Solid Edge part; units mm, degrees
sketch "Sketch1" plane through (0, 0, 0) normal (1, 0, 0) x (0, 1, 0)
  line L0 (0, 0) -> (43.8289, 0)
sketch "Sketch2" plane through (0, 0, 0) normal (0, -1, 0) x (1, 0, 0)
  line L0 (0, 50.8) -> (0, 0)
  line L1 (0, 0) -> (50.8, 0)
  line L2 (50.8, 0) -> (50.8, 6.35)
  line L3 (50.8, 6.35) -> (6.35, 6.35)
  line L4 (6.35, 6.35) -> (6.35, 50.8)
  line L5 (6.35, 50.8) -> (0, 50.8)
sweep "SweptProtrusion_1" add profiles "Sketch2" path "Sketch1"
Could you check a few things on this model? Use its own coordinates, in mm. A direction names the side the tool comes from. Round coordinates to 2 decimals unless told otherwise and drop trailing zeros. Loops run counter-clockwise (first coordinate to the right, second up) from the corner with the lowest first, then second, coordinate; pieces in that order, holes last.
Q1. I want a section at B-B (y = 3.5). Write out the boundary of the cut face in (x, z).
Q2. I want a section at C-C (z = 48). Write out the boundary of the cut face in (x, y), and give its area (3 significant figures).
Q3. Please list where this line runs through material, in increasing order: L1, parallel to X at y = 5.5, z = 29.
Q4. I want a section at A-A (x = 8.5). Write out the boundary of the cut face in (y, z), and give its area (3 significant figures).
Q5. On a 3-axis mill with a long thin cutter (end or side, diameter ignored), from which of +Z, -Z, +X, -X, +Y, -Y can I reach the whole of each face in a straight line? I mean faces 1 (the flat face through (3, 22, 50.8)), 2 (the flat face through (29, 22, 6.35)). Say none if no direction works.
Q6. For P1, Ø6, axis at x = 36, y = 17.5, coming from the +Z side; P2, Ø2, axis at y = 6, z = 42, coming from the +X side, each with a flat end and sliding along its axis, tell me the tip position at first contact or that it passes through.
Answer below:
1. outline: (0, 0) - (50.8, 0) - (50.8, 6.35) - (6.35, 6.35) - (6.35, 50.8) - (0, 50.8) - close
2. outline: (0, 0) - (6.35, 0) - (6.35, 43.83) - (0, 43.83) - close
2. area: 278 mm2
3. L1: x = 0 to 6.35
4. outline: (0, 0) - (43.83, 0) - (43.83, 6.35) - (0, 6.35) - close
4. area: 278 mm2
5. face 1: +Z, +X, -X, +Y, -Y
5. face 2: +Z, +X, +Y, -Y
6. P1: stops at z = 6.35
6. P2: stops at x = 6.35
